Autodesk Inventor part; units mm, degrees
ref_plane "YZ Plane" through (0, 0, 0) normal (1, 0, 0) x (0, 1, 0)
ref_plane "XZ Plane" through (0, 0, 0) normal (0, 1, 0) x (-1, 0, 0)
ref_plane "XY Plane" through (0, 0, 0) normal (0, 0, 1) x (1, 0, 0)
sketch "Эскиз1" plane through (0, 0, 0) normal (0, 1, 0) x (-1, 0, 0)
  line L0 (0, 0) -> (0, -39)
  line L1 (0, -39) -> (8, -39)
  line L2 (8, -39) -> (8, 0)
  line L3 (8, 0) -> (8, -19.75)
  line L4 (8, -19.75) -> (11, -19.75)
  line L5 (11, -19.75) -> (11, 0)
  line L6 (11, 0) -> (11, -20)
  line L7 (11, -20) -> (35, -20)
  line L8 (35, -20) -> (35, 0)
  line L9 (35, 0) -> (35, -12)
  line L10 (35, -12) -> (0, -12)
  line L11 (0, 0) -> (35, 0)
  line L12 (8, -19.75) -> (8, -20.75)
  line L13 (8, -20.75) -> (9, -20.75)
  circle A0 centre (9, -20.75) radius 1
  line L14 (11, -20) -> (9, -19.75)
  point P0 (9.2462, -19.7808)
  dimension "d0" = 39
  dimension "d1" = 8
  dimension "d2" = 19.75
  dimension "d3" = 3
  dimension "d4" = 20
  dimension "d6" = 12
  dimension "d27" = 1
  dimension "d28" = 1
revolve "Вращение1" add sketch "Эскиз1" angle 360 about axis through (0, 0, 0) along (-1, 0, 0) contours L10 L2 L1 L0 | L10 L5 L4 L2 | L10 L8 L7 L6 L5
sketch "Эскиз2" plane through (0, 0, 0) normal (1, 0, 0) x (0, 0, -1)
  line L0 (25, -16) -> (-25, -16)
  line L1 (-25, -16) -> (-25, 16)
  line L2 (-25, 16) -> (25, 16)
  line L3 (25, 16) -> (25, -16)
  line L4 (25, -16) -> (-25, 16) construction
  line L5 (-25, -16) -> (25, 16) construction
  line L6 (0, 0) -> (0, -27.5)
  line L7 (0, -27.5) -> (39.6722, -27.5)
  line L8 (39.6722, -27.5) -> (-36.2697, -27.5)
  line L9 (0, 0) -> (0, 27.5)
  line L10 (0, 27.5) -> (-39.8646, 27.5)
  line L11 (-39.8646, 27.5) -> (34.879, 27.5)
  circle A0 centre (0, 0) radius 39
  point P0 (27.6541, 27.5)
  point P1 (-27.6541, 27.5)
  point P2 (-27.6541, -27.5)
  point P3 (27.6541, -27.5)
  dimension "d8" = 50
  dimension "d9" = 32
  dimension "d23" = 27.5
  dimension "d24" = 27.5
hole "Отверстие1" at (0, -16, 25) at (0, 16, 25) at (0, 16, -25) at (0, -16, -25) direction (-1, 0, 0) diameter 9 end through all
chamfer "Фаска1" distance 2 angle 45 1 edges at (-35, 0, 20)
chamfer "Фаска2" distance 3 angle 45 1 edges at (-35, 0, 12)
extrude "Выдавливание1" cut sketch "Эскиз2" against normal through all contours L7 A0 L8 | L10 A0 L11
revolve "Вращение2" add sketch "Эскиз1" angle 360 about axis through (0, 0, 0) along (-1, 0, 0) contours L4 A0 L2 | L4 L6 L14 A0
thread "Резьба1"
properties part number "Втулка-4"
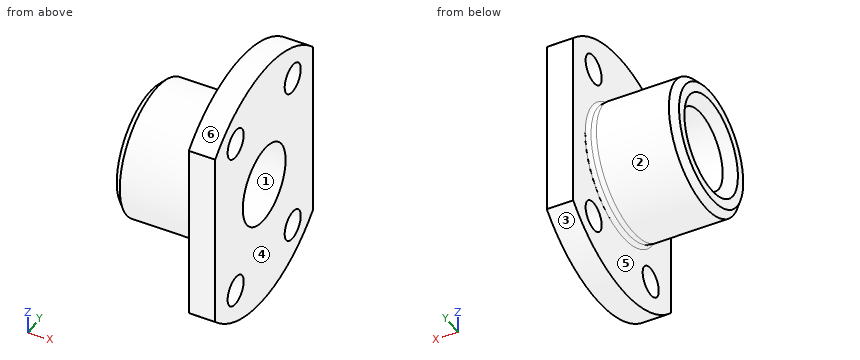
Here's how the part is built. I have some questions about the finished solid (model axes, mm). Face numbers are marked on the shaded views. A direction names the side the tool comes from. Give positions to 0.01 mm unless a question says otherwise; leave off trailing zeros. Order: outer loops, then holes, each group sorted by start corner. A loop starts at its lowest first (then second) coordinate and runs counter-clockwise, first axis right, second up. Notation, with made-up numbers: M 58,-23.5 L 98,-23.5 A18 ccw 98,-1.5 Z; hole C 66.5,68.25 d6. An arc over 180 degrees is marked long. Use a Markdown table: item, result. Add a question column.
1. If we mould it in two halves opening along Z, with no side actions, what happens to the marked faces 1, 2, 3 and 4? For each: +Z half, -Z half, draft (parallel to the pull), parting line (faces both ways), or undercut.
2. Suppose I cut it at C-C (z = 0). List the corners of the cut face in (x, y) for me, and give its area (3 significant figures).
3. I need wall thicknesses on probe 1 along Y at (x, z) = (-3, -25); probe 2 along Z at (x, y) = (-2.25, -16); probe 3 along X at (y, z) = (-4, 27.5). Which ranges of each line are inside material? Lowest first, please. Write a range as from..to.
4. On a 3-axis mill with a long thin cutter (end or side, diameter ignored), from which of +Z, -Z, +X, -X, +Y, -Y can I reach the whole of each face in a straight line? I mean the marked faces 5 and 6. Say none if no direction works.
5. Suppose I cut it at B-B (y = 0). List the corners of the cut face in (x, z) for me.
6. Suppose I cut it at A-A (z = -25). List the corners of the cut face in (x, y) for me, and give its area (3 significant figures).
7. Suppose I cut it at D-D (x = -22.5). List the corners of the cut face in (y, z) for me, and give its area (3 significant figures).
8. For pin 1 Ø14.5 at (y, z) = (-16, 25) entering from -X; pin 2 Ø8 at (x, y) = (-16, 10.5) entering from -Z; pin 3 Ø7 at (y, z) = (16, 25) entering from -X; pin 4 Ø3 at (x, z) = (-10.5, -2) entering from -Y, each with a flat end and sliding along its axis, tell me the tip position at first contact or that it passes through.
Results list:
| question | item | result |
|---|---|---|
| 1 | face 1 | undercut |
| 1 | face 2 | parting line |
| 1 | face 3 | -Z half |
| 1 | face 4 | draft |
| 2 | outline | M -35,-18 L -33,-20 L -11,-20 L -9.25,-19.78 A1 cw -8,-20.75 L -8,-27.5 L 0,-27.5 L 0,-12 L -32,-12 L -35,-15 Z; M -35,15 L -32,12 L 0,12 L 0,27.5 L -8,27.5 L -8,20.75 A1 cw -9.25,19.78 L -11,20 L -33,20 L -35,18 Z |
| 2 | area | 666 mm² |
| 3 | probe 1 | y = -27.5..-20.5, -11.5..11.5, 20.5..27.5 |
| 3 | probe 2 | z = -35.57..-29.5, -20.5..20.5, 29.5..35.57 |
| 3 | probe 3 | x = -8..0 |
| 4 | face 5 | -X |
| 4 | face 6 | +Z, +X, -X |
| 5 | outline | M -35,-18 L -33,-20 L -11,-20 L -9.25,-19.78 A1 cw -8,-20.75 L -8,-39 L 0,-39 L 0,-12 L -32,-12 L -35,-15 Z; M -35,15 L -32,12 L 0,12 L 0,39 L -8,39 L -8,20.75 A1 cw -9.25,19.78 L -11,20 L -33,20 L -35,18 Z |
| 6 | outline | M -8,-27.5 L 0,-27.5 L 0,-20.5 L -8,-20.5 Z; M -8,-11.5 L 0,-11.5 L 0,11.5 L -8,11.5 Z; M -8,20.5 L 0,20.5 L 0,27.5 L -8,27.5 Z |
| 6 | area | 296 mm² |
| 7 | outline | C 0,0 d40; hole C 0,0 d24 |
| 7 | area | 804 mm² |
| 8 | pin 1 | stops at x = -8 |
| 8 | pin 2 | stops at z = -18.91 |
| 8 | pin 3 | passes through |
| 8 | pin 4 | stops at y = -19.99 |
